Read the model definition and answer for the solid it produces. Units are mm, in the model's axes. A direction names the side the tool comes from. Coordinates: 2 decimals unless noted, no trailing zeros. Order: outer loops, then holes, each group sorted by start corner. A loop starts at its lowest first (then second) coordinate and runs counter-clockwise, first axis right, second up. Notation, with made-up numbers: (62.5, 59) -> (91.5, 59) arc R20 ccw to (91.5, 81) -> close; hole circle Ø5 at (-2.75, 80). An arc over 180 degrees is marked (long way). Answer as a JSON object with one key per item and string values. Group by question number.
1) Given pin 1 (1 mm diameter, centred on x = -13, y = 9.5, fed in from -Z); pin 2 (15 mm diameter, centred on y = 15, z = -13.5, fed in from +X); pin 3 (8 mm diameter, centred on x = -10.5, y = 22.5, fed in from +Z), each flat-ended and moving along its own axis, determine where each tip first touches the part or whether it passes through.
2) Consider L1, parallel to Y at x = -16.75, z = -3.5; L2, parallel to Z at x = -4.25, y = 33; L3, parallel to X at y = 34, z = -16.75. Determine where each line is inside the solid, lowest interval first.
3) Section A-A on x = -14 is taken. Determine the outline of the cut face in (y, z).
4) Section B-B on z = -2.75 is taken. Determine the outline of the cut face in (x, y), and give its area (3 significant figures).
5) A tool of negligible diameter and unlimited length cuts with its end or side. For faces 1 (the flat face through (0, 20, -9)), 2 (the flat face through (-8, 20, -18.7)), 3 (the flat face through (-15.7, 20, -9)), 4 (the flat face through (-8, 20, 0)), from which of +Z, -Z, +X, -X, +Y, -Y can it reach the whole face along a straight path? Write none if from no direction.
6) Section D-D on z = -20.75 is taken. Determine the outline of the cut face in (x, y).
7) Section C-C on y = 10 is taken. Determine the outline of the cut face in (x, z), and give its area (3 significant figures).
Autodesk Inventor part; units mm, degrees
ref_plane "YZ Plane" through (0, 0, 0) normal (1, 0, 0) x (0, 1, 0)
ref_plane "XZ Plane" through (0, 0, 0) normal (0, 1, 0) x (-1, 0, 0)
ref_plane "XY Plane" through (0, 0, 0) normal (0, 0, 1) x (1, 0, 0)
sketch "Sketch1" plane through (0, 0, 0) normal (0, 1, 0) x (-1, 0, 0)
  line L0 (0, 0) -> (0, -18.7)
  line L1 (0, -18.7) -> (0, -11.8708)
  line L2 (0, -18.7) -> (15.7, -18.7)
  line L3 (15.7, -18.7) -> (15.7, 0)
  line L4 (15.7, 0) -> (0, 0)
  dimension "d0" = 18.7
  dimension "d1" = 15.7
extrude "Extrusion1" add sketch "Sketch1" along normal blind 40.5
sketch "Sketch2" plane through (0, 40.5, 0) normal (0, 1, 0) x (1, 0, 0)
  line L0 (0, 0) -> (0, 18.7)
  line L1 (0, 18.7) -> (0, 23.7)
  line L2 (0, 23.7) -> (-15.7, 23.7)
  line L3 (-15.7, 23.7) -> (-20.7, 23.7)
  line L4 (-20.7, 23.7) -> (-20.7, 0)
  line L5 (-20.7, 0) -> (-20.7, -5)
  line L6 (-20.7, -5) -> (0, -5)
  line L7 (0, -5) -> (5, -5)
  line L8 (5, -5) -> (5, 18.7)
  line L9 (5, 18.7) -> (5, 23.7)
  line L10 (0, 23.7) -> (5, 23.7)
  dimension "d4" = 5
  dimension "d5" = 5
  dimension "d6" = 5
  dimension "d7" = 5
extrude "Extrusion2" add sketch "Sketch2" along normal blind 5
properties part number "chaveta"
Worked answers:
{
 "1": {"pin 1": "stops at z = -18.7", "pin 2": "stops at x = 0", "pin 3": "stops at z = 0"},
 "2": {"L1": "y = 40.5 to 45.5", "L2": "z = -18.7 to 0", "L3": "x = -15.7 to 0"},
 "3": {"outline": "(0, -18.7) -> (40.5, -18.7) -> (40.5, -23.7) -> (45.5, -23.7) -> (45.5, 5) -> (40.5, 5) -> (40.5, 0) -> (0, 0) -> close"},
 "4": {"outline": "(-20.7, 40.5) -> (-15.7, 40.5) -> (-15.7, 0) -> (0, 0) -> (0, 40.5) -> (5, 40.5) -> (5, 45.5) -> (-20.7, 45.5) -> close", "area": "764 mm²"},
 "5": {"face 1": "+Z, -Z, +X, -Y", "face 2": "-Z, +X, -X, -Y", "face 3": "+Z, -Z, -X, -Y", "face 4": "+Z, +X, -X, -Y"},
 "6": {"outline": "(-20.7, 40.5) -> (5, 40.5) -> (5, 45.5) -> (-20.7, 45.5) -> close"},
 "7": {"outline": "(-15.7, -18.7) -> (0, -18.7) -> (0, 0) -> (-15.7, 0) -> close", "area": "294 mm²"}
}
